from build123d import *

# Parameters (mm, degrees)
F0_R       = 3.25
F0_R_2     = 2.9
F0_R_3     = 1.25
F1_DEPTH   = 5
F2_SIZE2   = 2.2392304845
F2_SIZE    = 0.6
F2_2_SIZE2 = 2.2392304845
F2_2_SIZE  = 0.6


with BuildPart() as f1:
    # F0 (on Top) → F1 (new body)
    with BuildSketch(Plane.XY):
        Circle(F0_R)
        Circle(F0_R_2, mode=Mode.SUBTRACT)
        Circle(F0_R_2)
        Circle(F0_R_3, mode=Mode.SUBTRACT)
    extrude(amount=F1_DEPTH)

    # F2
    f2_edges = [f1.edges().sort_by_distance(p)[0] for p in [
        (-3.25, 0, 5),
    ]]
    f2_side = f1.faces().sort_by_distance((-1.341924, 0, 5))[0]
    chamfer(f2_edges, length=F2_SIZE, length2=F2_SIZE2, reference=f2_side)

    # F2#2
    f2_2_edges = [f1.edges().sort_by_distance(p)[0] for p in [
        (-3.25, 0, 0),
    ]]
    f2_2_side = f1.faces().sort_by_distance((-1.341924, 0, 0))[0]
    chamfer(f2_2_edges, length=F2_2_SIZE, length2=F2_2_SIZE2, reference=f2_2_side)


solid = f1.part
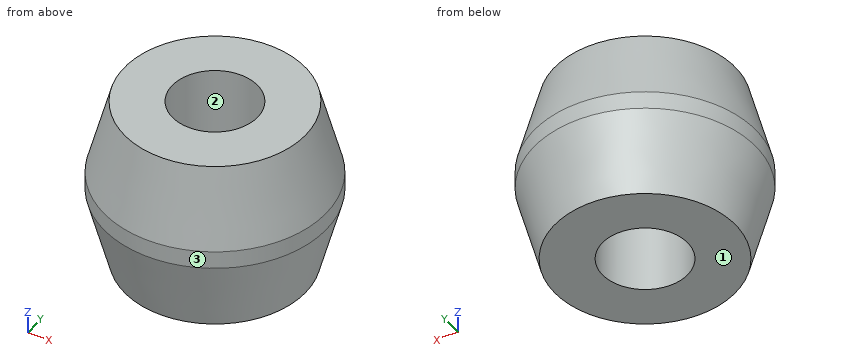
Geometry check sheet. Reference: the model listing, model coordinates, mm. Face numbers are marked on the shaded views. Round coordinates to 2 decimals unless told otherwise and drop trailing zeros. Order: outer loops, then holes, each group sorted by start corner. A loop starts at its lowest first (then second) coordinate and runs counter-clockwise, first axis right, second up. Notation, with made-up numbers: M -40,22 L -19,22 A30 ccw -19,50 Z; hole C -10.5,71 d10. An arc over 180 degrees is marked long. Answer in a Markdown table with one row per item. Add a question column.
Item 1: Material ranges on L1, parallel to Y at x = 0, z = 2.6; L2, parallel to X at y = 1, z = 4.6; L3, parallel to X at y = -0.5, z = 3.9, recorded low to high. Write a range as [from, to].
Item 2: Draft check along Y on the marked faces 1, 2 and 3. Enter one of: released by +Y, released by -Y, zero draft, split by the parting line, or undercut.
Item 3: Sectioned sample at C-C, the plane z = 0.8. Enter the section's corners in (x, y), plus the area to 3 significant figures.
Item 4: Depth check by flat-ended pin: pin 1 Ø2 at (y, z) = (-0.5, 4.5) entering from -X; pin 2 Ø3 at (x, z) = (0, 3) entering from -Y; pin 3 Ø1 at (x, y) = (0, 0.5) entering from +Z. Enter the tip coordinate at first touch or a pass-through.
Item 5: Sectioned sample at A-A, the plane y = 0. Enter the section's corners in (x, z).
Item 6: Sectioned sample at D-D, the plane z = 4.6. Enter the section's corners in (x, y).
Filled in:
| question | item | result |
|---|---|---|
| 1 | L1 | y = [-3.25, -1.25], [1.25, 3.25] |
| 1 | L2 | x = [-2.57, -0.75], [0.75, 2.57] |
| 1 | L3 | x = [-2.9, -1.15], [1.15, 2.9] |
| 2 | face 1 | zero draft |
| 2 | face 2 | undercut |
| 2 | face 3 | split by the parting line |
| 3 | outline | C 0,0 d5.73; hole C 0,0 d2.5 |
| 3 | area | 20.9 mm² |
| 4 | pin 1 | stops at x = -3.03 |
| 4 | pin 2 | stops at y = -3.25 |
| 4 | pin 3 | passes through |
| 5 | outline | M -3.25,2.24 L -2.65,0 L -1.25,0 L -1.25,5 L -2.65,5 L -3.25,2.76 Z; M 1.25,0 L 2.65,0 L 3.25,2.24 L 3.25,2.76 L 2.65,5 L 1.25,5 Z |
| 6 | outline | C 0,0 d5.51; hole C 0,0 d2.5 |
